CAD build for the part. Positions are in the model's coordinates, mm. Give positions to 0.01 mm unless a question says otherwise; leave off trailing zeros. Write each loop counter-clockwise with the first axis right and the second up, starting at its lowest first coordinate (ties: lowest second). Pieces come first, ordered by that corner, then holes. Notation, with made-up numbers: (20.25, 23) - (69.25, 23) arc R20 ccw to (69.25, 33) - close; hole circle Ø6 at (50, 26.25). An arc over 180 degrees is marked (long way). Put each result on its own line as item: value. Start each with the question number.
1. Cut at A-A on y = -1.8. Give the number of separate pieces and of enclosed holes in the cut face, and give its area (3 significant figures).
2. Cut at C-C on x = 43. List the corners of the cut face in (y, z).
3. Cut at B-B on z = 95.25. List the corners of the cut face in (x, y).
4. Drop flat-ended pins along their axis: pin 1 (5.5 mm diameter, centred on x = 0, z = 0, fed in from -Y); pin 2 (1 mm diameter, centred on x = 46.5, y = -1, fed in from +Z). Give the stop position or say it passes through.
5. Wall check: line 1 (X direction, y = -1.3, z = -1); line 2 (Z direction, x = 2, y = -1.05); line 3 (X direction, y = -1, z = 90.5). Give the ranges that are in metal, low to high.
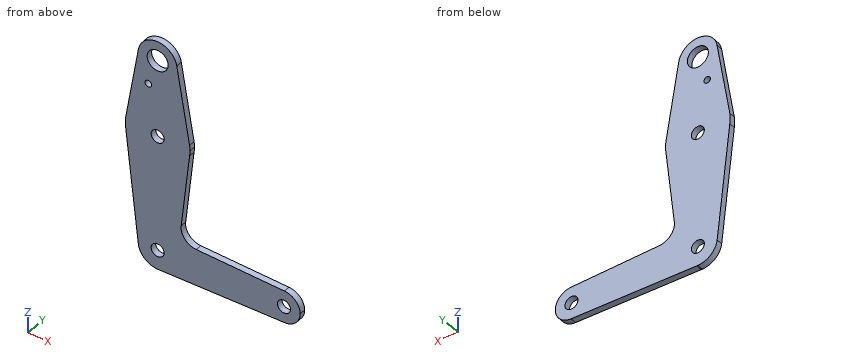
from build123d import *

# Parameters (mm, degrees)
F0_R     = 5.139884
F0_R_2   = 1.5875
F0_R_3   = 3.175
F0_R_4   = 3.174261
F1_DEPTH = 3.048


with BuildPart() as f1:
    # F0 (on Front) → F1 (new body)
    with BuildSketch(Plane.XZ):
        with BuildLine():
            ThreePointArc((-9.391777, 96.8375), (-0.79654, 85.758364), (9.525, 95.25))
            ThreePointArc((9.525, 95.25), (9.491636, 96.04654), (9.391777, 96.8375))
            ThreePointArc((9.391777, 96.8375), (0, 104.775), (-9.391777, 96.8375))
        make_face()
        with Locations((0, 95.25)):
            Circle(F0_R, mode=Mode.SUBTRACT)
        with BuildLine():
            ThreePointArc((9.391777, 96.8375), (9.491636, 96.04654), (9.525, 95.25))
            ThreePointArc((9.525, 95.25), (-0.79654, 85.758364), (-9.391777, 96.8375))
            Line((-9.391777, 96.8375), (-15.652961, 59.795833))
            ThreePointArc((-15.652961, 59.795833), (0, 73.025), (15.652961, 59.795833))
            Line((15.652961, 59.795833), (9.391777, 96.8375))
        make_face()
        with Locations((-4.567989, 81.601493)):
            Circle(F0_R_2, mode=Mode.SUBTRACT)
        with BuildLine():
            ThreePointArc((15.875, 57.15), (15.819393, 58.477567), (15.652961, 59.795833))
            ThreePointArc((15.652961, 59.795833), (0, 73.025), (-15.652961, 59.795833))
            ThreePointArc((-15.652961, 59.795833), (-15.875, 57.15), (-15.652961, 54.504167))
            ThreePointArc((-15.652961, 54.504167), (0, 41.275), (15.652961, 54.504167))
            ThreePointArc((15.652961, 54.504167), (15.819393, 55.822433), (15.875, 57.15))
        make_face()
        with Locations((0, 57.15)):
            Circle(F0_R_3, mode=Mode.SUBTRACT)
        with BuildLine():
            ThreePointArc((15.652961, 54.504167), (0, 41.275), (-15.652961, 54.504167))
            Line((-15.652961, 54.504167), (-9.466493, -1.054103))
            ThreePointArc((-9.466493, -1.054103), (-0.527863, 9.510362), (9.525, 0))
            ThreePointArc((9.525, 0), (6.905344, -6.560628), (0.487342, -9.512525))
            Line((0.487342, -9.512525), (62.115626, -7.934901))
            ThreePointArc((62.115626, -7.934901), (53.975, 0), (62.115626, 7.934901))
            Line((62.115626, 7.934901), (18.910892, 9.0409))
            ThreePointArc((18.910892, 9.0409), (13.362859, 11.650215), (11.532699, 17.501687))
            Line((11.532699, 17.501687), (15.652961, 54.504167))
        make_face()
        with BuildLine():
            ThreePointArc((9.525, 0), (-0.527863, 9.510362), (-9.466493, -1.054103))
            ThreePointArc((-9.466493, -1.054103), (-6.351586, -7.098097), (0, -9.525))
            Line((0, -9.525), (0.487342, -9.512525))
            ThreePointArc((0.487342, -9.512525), (6.905344, -6.560628), (9.525, 0))
        make_face()
        Circle(F0_R_4, mode=Mode.SUBTRACT)
        with BuildLine():
            Line((0.487342, -9.512525), (0, -9.525))
            ThreePointArc((0, -9.525), (0.243751, -9.521881), (0.487342, -9.512525))
        make_face()
        with BuildLine():
            ThreePointArc((69.85, 0), (67.596522, 5.540379), (62.115626, 7.934901))
            ThreePointArc((62.115626, 7.934901), (53.975, 0), (62.115626, -7.934901))
            ThreePointArc((62.115626, -7.934901), (67.596522, -5.540379), (69.85, 0))
        make_face()
        with Locations((61.9125, 0)):
            Circle(F0_R_3, mode=Mode.SUBTRACT)
    extrude(amount=F1_DEPTH)


solid = f1.part
Report:
1. separate pieces: 1
1. enclosed holes: 5
1. area: 3,570 mm²
2. outline: (-3.05, -8.42) - (0, -8.42) - (0, 8.42) - (-3.05, 8.42) - close
3. outline: (-9.66, -3.05) - (-5.14, -3.05) - (-5.14, 0) - (-9.66, 0) - close; (5.14, -3.05) - (9.66, -3.05) - (9.66, 0) - (5.14, 0) - close
4. pin 1: passes through
4. pin 2: stops at z = 8.35
5. line 1: x = -9.47 to -3.01, 3.01 to 58.9, 64.93 to 69.79
5. line 2: z = -9.47 to -2.46, 2.46 to 54.68, 59.62 to 90.52, 99.98 to 104.56
5. line 3: x = -10.46 to -1.96, 1.96 to 10.46
